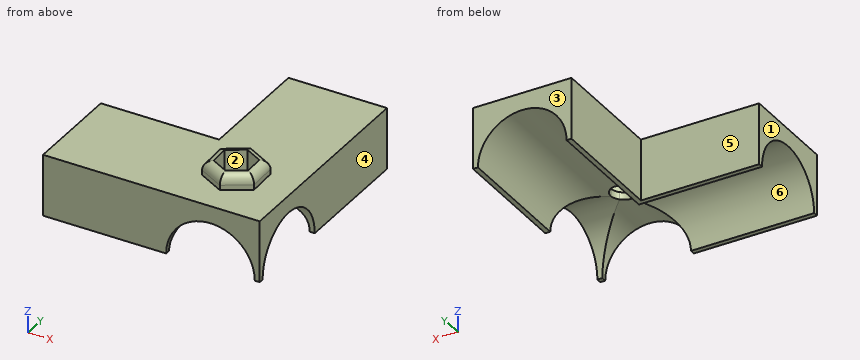
```python
from build123d import *

# Parameters (mm, degrees)
F1_DEPTH      = 25
F2_R          = 9
F3_DEPTH      = 44.001
F4_R          = 9
F5_DEPTH      = 44.001
F7_DEPTH      = 44.0010001
F8_R          = 2.5
F9_DEPTH      = 2
F10_DEPTH     = 3
F11_T1_DEPTH  = 16
F11_T3_DEPTH  = 16
F11_T5_DEPTH  = 16
F11_T7_DEPTH  = 16
F11_T9_DEPTH  = 16
F11_T11_DEPTH = 16


# Not quite as in the source:
# - a fillet or chamfer that OpenCascade refuses, or shapes differently, is made with other operations: its cross-section is extruded or revolved along the edge and cut away or added


with BuildPart() as f1:
    # F0 (on Top) → F1 (new body)
    with BuildSketch(Plane.XY):
        with BuildLine():
            Line((6.9382145885, -6.9382145885), (0, 0))
            Line((0, 0), (-24, 0))
            Line((-24, 0), (-24, -20))
            Line((-24, -20), (20, -20))
            Line((20, -20), (10.4737484944, -10.4737484944))
            ThreePointArc((10.4737484944, -10.4737484944), (6.9382145885, -10.4737484944), (6.9382145885, -6.9382145885))
        make_face()
        with BuildLine():
            Line((20, 24), (0, 24))
            Line((0, 24), (0, 0))
            Line((0, 0), (6.9382145885, -6.9382145885))
            ThreePointArc((6.9382145885, -6.9382145885), (9.6626901223, -6.3962827101), (11.2059815414, -8.7059815414))
            ThreePointArc((11.2059815414, -8.7059815414), (11.0156803727, -9.6626901223), (10.4737484944, -10.4737484944))
            Line((10.4737484944, -10.4737484944), (20, -20))
            Line((20, -20), (20, 24))
        make_face()
    extrude(amount=F1_DEPTH)

    # F2 (on face) → F3 (cut, through all)
    with BuildSketch(Plane(origin=(-24, 0, 0), x_dir=(0, -1, 0), z_dir=(-1, 0, 0))):
        with Locations((10, 12.5)):
            Circle(F2_R)
    extrude(amount=-F3_DEPTH, mode=Mode.SUBTRACT)

    # F4 (on face) → F5 (cut, through all)
    with BuildSketch(Plane(origin=(0, 24, 0), x_dir=(-1, 0, 0), z_dir=(0, 1, 0))):
        with Locations((-10, 12.5)):
            Circle(F4_R)
    extrude(amount=-F5_DEPTH, mode=Mode.SUBTRACT)

    # F6 (on face) → F7 (cut, through all)
    with BuildSketch(Plane.XZ.offset(20)):
        with BuildLine():
            Line((20, 12.5), (19, 12.5))
            ThreePointArc((19, 12.5), (10, 3.5), (1, 12.5))
            Line((1, 12.5), (-24, 12.5))
            Line((-24, 12.5), (-24, 0))
            Line((-24, 0), (20, 0))
            Line((20, 0), (20, 12.5))
        make_face()
    extrude(amount=-F7_DEPTH, mode=Mode.SUBTRACT)

    # F8 (on face) → F9 (cut)
    with BuildSketch(Plane.XY.offset(25)):
        Polygon((5.0551444558, -6.7069682099), (5.1807740761, -10.704994873), (8.7059815414, -12.5952097618), (12.1055593865, -10.4873979877), (11.9799297662, -6.4893713246), (8.4547223009, -4.5991564357), align=None)
        with Locations((8.7059815414, -8.7059815414)):
            Circle(F8_R, mode=Mode.SUBTRACT)
    extrude(amount=-F9_DEPTH, mode=Mode.SUBTRACT)

    # F8 (on face) → F10 (join)
    with BuildSketch(Plane.XY.offset(25)):
        Polygon((3.229725913, -5.7074615441), (3.4181703434, -11.7045015387), (8.7059815414, -14.5398238721), (13.805348309, -11.3781062108), (13.6169038786, -5.3810662162), (8.3290926806, -2.5457438829), align=None)
        Polygon((8.7059815414, -12.5952097618), (5.1807740761, -10.704994873), (5.0551444558, -6.7069682099), (8.4547223009, -4.5991564357), (11.9799297662, -6.4893713246), (12.1055593865, -10.4873979877), align=None, mode=Mode.SUBTRACT)
    extrude(amount=F10_DEPTH)

    # F11: fillet of radius 2 on 6 edges, made by hand

    # F11_s2 → F11_t1 (cut)
    with BuildSketch(Plane(origin=(17.2236751454, -9.2353279974, 0), x_dir=(0, 0, 1), z_dir=(-0.8813018663, 0.4725537222, 0))):
        with BuildLine():
            ThreePointArc((26, 1.6923749137), (27.4142135624, 1.1065884761), (28, -0.3076250863))
            Line((28, -0.3076250863), (28, 1.6923749137))
            Line((28, 1.6923749137), (26, 1.6923749137))
        make_face()
    extrude(amount=F11_T1_DEPTH, mode=Mode.SUBTRACT)

    # F11_s4 → F11_t3 (cut)
    with BuildSketch(Plane(origin=(0.5278354617, -16.7977921518, 0), x_dir=(0, 0, 1), z_dir=(-0.0314074051, 0.9995066658, 0))):
        with BuildLine():
            ThreePointArc((28, 11.4411808674), (27.4142135624, 12.8553944297), (26, 13.4411808674))
            Line((26, 13.4411808674), (28, 13.4411808674))
            Line((28, 13.4411808674), (28, 11.4411808674))
        make_face()
    extrude(amount=F11_T3_DEPTH, mode=Mode.SUBTRACT)

    # F11_s6 → F11_t5 (cut)
    with BuildSketch(Plane(origin=(-4.4726864595, -2.7731623193, 0), x_dir=(0, 0, 1), z_dir=(0.8498944613, 0.5269529435, 0))):
        with BuildLine():
            ThreePointArc((28, 14.9449583763), (27.4142135624, 16.3591719387), (26, 16.9449583763))
            Line((26, 16.9449583763), (28, 16.9449583763))
            Line((28, 16.9449583763), (28, 14.9449583763))
        make_face()
    extrude(amount=F11_T5_DEPTH, mode=Mode.SUBTRACT)

    # F11_s8 → F11_t7 (cut)
    with BuildSketch(Plane(origin=(3.122845284, -1.6744684418, 0), x_dir=(0, 0, 1), z_dir=(0.8813018663, -0.4725537222, 0))):
        with BuildLine():
            ThreePointArc((28, 6.6999299317), (27.4142135624, 8.1141434941), (26, 8.6999299317))
            Line((26, 8.6999299317), (28, 8.6999299317))
            Line((28, 8.6999299317), (28, 6.6999299317))
        make_face()
    extrude(amount=F11_T7_DEPTH, mode=Mode.SUBTRACT)

    # F11_s10 → F11_t9 (cut)
    with BuildSketch(Plane(origin=(0.0253169806, -0.8056854995, 0), x_dir=(0, 0, 1), z_dir=(0.0314074051, -0.9995066658, 0))):
        with BuildLine():
            ThreePointArc((28, -5.048876022), (27.4142135624, -3.6346624596), (26, -3.048876022))
            Line((26, -3.048876022), (28, -3.048876022))
            Line((28, -3.048876022), (28, -5.048876022))
        make_face()
    extrude(amount=F11_T9_DEPTH, mode=Mode.SUBTRACT)

    # F11_s12 → F11_t11 (cut)
    with BuildSketch(Plane(origin=(9.1256249208, 5.6580847774, 0), x_dir=(0, 0, 1), z_dir=(-0.8498944613, -0.5269529435, 0))):
        with BuildLine():
            ThreePointArc((28, -8.5526535309), (27.4142135624, -7.1384399686), (26, -6.5526535309))
            Line((26, -6.5526535309), (28, -6.5526535309))
            Line((28, -6.5526535309), (28, -8.5526535309))
        make_face()
    extrude(amount=F11_T11_DEPTH, mode=Mode.SUBTRACT)


solid = f1.part
```
Read the model definition and answer for the solid it produces. Units are mm, in the model's axes. Face numbers are marked on the shaded views. A direction names the side the tool comes from. Coordinates: 2 decimals unless noted, no trailing zeros. Write each loop counter-clockwise with the first axis right and the second up, starting at its lowest first coordinate (ties: lowest second). Pieces come first, ordered by that corner, then holes. Notation, with made-up numbers: (39, 32.25) -> (80, 32.25) arc R23 cw to (80, 56.25) -> close; hole circle Ø2 at (68, -24.75). An arc over 180 degrees is marked (long way). Write item = value, one per line.
(1) Straight lines are drawn through the part: L1, parallel to Y at x = 17.5, z = 20; L2, parallel to Y at x = -2.5, z = 20.25; L3, parallel to X at y = 1.5, z = 22. For each, find the intervals that lie inside material, in ascending order. Write a range as from..to.
From the geometry:
L1 = -20..-14.97, -5.03..24
L2 = -20..-14.58, -5.42..0
L3 = 0..20
(2) Given pin 1 Ø1 at (x, y) = (-3.5, -2.5) entering from -Z; pin 2 Ø1.5 at (x, y) = (15.5, -2.5) entering from -Z; pin 3 Ø2 at (x, y) = (7, -7.5) entering from +Z, each flat-ended and moving along its own axis, determine where each tip first touches the part or whether it passes through.
From the geometry:
pin_1 = 16.62
pin_2 = 18.98
pin_3 = 23
(3) For a pull along X with two mould halves and no side action, classify the marked faces 1, 2, 3 and 4 as +X half, -X half, draft (parallel to the pull), parting line (faces both ways), or undercut.
From the geometry:
face_1 = -X half
face_2 = undercut
face_3 = draft
face_4 = +X half
(4) Section A-A on z = 24.25 is taken. Write down the section's boundary in (x, y) (3 decimals).
From the geometry:
outline = (-24, -20) -> (20, -20) -> (20, 24) -> (0, 24) -> (0, 0) -> (-24, 0) -> close; hole (5.055, -6.707) -> (5.181, -10.705) -> (8.706, -12.595) -> (12.106, -10.487) -> (11.98, -6.489) -> (8.455, -4.599) -> close
(5) Which of the six approach directions +Z, -Z, +X, -X, +Y, -Y give full straight-line access (tool end or side, diameter ignored) to the marked faces 5 and 6?
From the geometry:
face_5 = +Z, -Z, -X, +Y
face_6 = -Z, +X, -X
(6) Section C-C on x = -1 is taken. Write down the section's boundary in (y, z), plus the area to 3 significant figures.
From the geometry:
outline = (-20, 12.5) -> (-19, 12.5) arc R9 cw to (-1, 12.5) -> (0, 12.5) -> (0, 25) -> (-20, 25) -> close
area = 123 mm2
(7) Section D-D on y = 16 is taken. Write down the section's boundary in (x, z).
From the geometry:
outline = (0, 12.5) -> (1, 12.5) arc R9 cw to (19, 12.5) -> (20, 12.5) -> (20, 25) -> (0, 25) -> close
(8) Section B-B on z = 14.5 is taken. Write down the section's boundary in (x, y).
From the geometry:
outline = (-24, -20) -> (1.23, -20) -> (1.23, -18.77) -> (-24, -18.77) -> close; (-24, -1.23) -> (1.23, -1.23) -> (1.23, 24) -> (0, 24) -> (0, 0) -> (-24, 0) -> close; (18.77, -20) -> (20, -20) -> (20, -18.77) -> (18.77, -18.77) -> close; (18.77, -1.23) -> (20, -1.23) -> (20, 24) -> (18.77, 24) -> close
